from build123d import *

# Parameters (mm, degrees)
SKETCH_W        = 50
SKETCH_H        = 50
PAD_DEPTH       = 25
FILLET_R        = 3
POCKET_DEPTH    = 20
SKETCH008_W     = 44.5
SKETCH008_H     = 40.5
POCKET001_DEPTH = 4
SKETCH009_W     = 40
SKETCH009_H     = 40
POCKET002_DEPTH = 1


with BuildPart() as part:
    # Sketch → Pad (new body)
    with BuildSketch(Plane.XY):
        Rectangle(SKETCH_W, SKETCH_H)
    extrude(amount=PAD_DEPTH)

    # Fillet
    fillet_edges = [part.edges().sort_by_distance(p)[0] for p in [
        (0, -25, 0),
        (-25, 0, 0),
        (0, 25, 0),
        (25, 0, 0),
        (-25, -25, 12.5),
        (25, 25, 12.5),
        (-25, 25, 12.5),
        (25, -25, 12.5),
    ]]
    fillet(fillet_edges, radius=FILLET_R)

    # Sketch007 (on Face2 of Fillet) → Pocket (cut)
    with BuildSketch(Plane.XY.offset(25)):
        Polygon((-20, 25), (-20, 24), (-22.25, 24), (-22.25, 22.3), (-20, 22.3), (-20, 20), (-22.3, 20), (-22.3, 22.25), (-24, 22.25), (-24, 20), (-25, 20), (-25, -20), (-24, -20), (-24, -22.25), (-22.3, -22.25), (-22.3, -20), (-20, -20), (-20, -22.3), (-22.25, -22.3), (-22.25, -24), (-20, -24), (-20, -25), (20, -25), (20, -24), (22.25, -24), (22.25, -22.3), (20, -22.3), (20, -20), (22.3, -20), (22.3, -22.25), (24, -22.25), (24, -20), (25, -20), (25, 20), (24, 20), (24, 22.25), (22.3, 22.25), (22.3, 20), (20, 20), (20, 22.3), (22.25, 22.3), (22.25, 24), (20, 24), (20, 25), align=None)
    extrude(amount=-POCKET_DEPTH, mode=Mode.SUBTRACT)

    # Sketch008 (on Face7 of Pocket) → Pocket001 (cut)
    with BuildSketch(Plane.XY.offset(5)):
        Rectangle(SKETCH008_W, SKETCH008_H)
    extrude(amount=-POCKET001_DEPTH, mode=Mode.SUBTRACT)

    # Sketch009 (on Face49 of Pocket001) → Pocket002 (cut)
    with BuildSketch(Plane.XY.offset(1)):
        Rectangle(SKETCH009_W, SKETCH009_H)
    extrude(amount=-POCKET002_DEPTH, mode=Mode.SUBTRACT)


solid = part.part
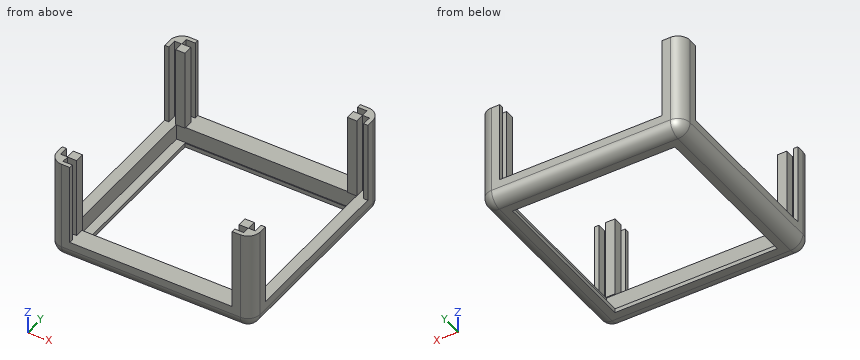
Input: part model. Units: mm. Frame: model coordinates. Round coordinates to 2 decimals unless told otherwise and drop trailing zeros. Write each loop counter-clockwise with the first axis right and the second up, starting at its lowest first coordinate (ties: lowest second). Pieces come first, ordered by that corner, then holes.
1) Cut plane D-D (y = -21). Return the cut outline in (x, z).
2) Contact query for flat-ended pins moving along their axis: P1, Ø2, axis at x = 23.5, y = -4, coming from the +Z side; P2, Ø0.5, axis at y = 0, z = 0.5, coming from the -X side; P3, Ø0.8, axis at x = 23, z = 19, coming from the -Y side. Output: stop coordinate, or through.
3) Cut plane A-A (x = 10). Return the cut outline in (y, z), then the cut area to 3 significant figures.
4) Cut plane C-C (z = 5.75). Count the separate pieces of the cut face and the enclosed holes in it, then the cut area to 3 significant figures.
5) Cut plane B-B (y = 6). Return the cut outline in (x, z).
6) Ray query, L1, parallel to X at y = 22, z = 19.5; L2, parallel to X at y = 17.5, z = 4; L3, parallel to Y at x = 5, z = 4.5. Return the intervals inside material, ascending.
Geometry says:
1. outline: (-25, 3) arc R3 ccw to (-22, 0) - (22, 0) arc R3 ccw to (25, 3) - (25, 25) - (24, 25) - (24, 5) - (22.3, 5) - (22.3, 25) - (20, 25) - (20, 5) - (-20, 5) - (-20, 25) - (-22.3, 25) - (-22.3, 5) - (-24, 5) - (-24, 25) - (-25, 25) - close
2. P1: stops at z = 5
2. P2: stops at x = -23.98
2. P3: stops at y = -24.94
3. outline: (-25, 3) arc R3 ccw to (-22, 0) - (-20, 0) - (-20, 1) - (-20.25, 1) - (-20.25, 5) - (-25, 5) - close; (20, 0) - (22, 0) arc R3 ccw to (25, 3) - (25, 5) - (20.25, 5) - (20.25, 1) - (20, 1) - close
3. area: 44.1 mm2
4. separate pieces: 4
4. enclosed holes: 0
4. area: 61.7 mm2
5. outline: (-25, 3) arc R3 ccw to (-22, 0) - (-20, 0) - (-20, 1) - (-22.25, 1) - (-22.25, 5) - (-25, 5) - close; (20, 0) - (22, 0) arc R3 ccw to (25, 3) - (25, 5) - (22.25, 5) - (22.25, 1) - (20, 1) - close
6. L1: x = -25 to -24, -22.3 to -20, 20 to 22.3, 24 to 25
6. L2: x = -25 to -22.25, 22.25 to 25
6. L3: y = -25 to -20.25, 20.25 to 25
